from build123d import *

# Parameters (mm, degrees)
SKETCH_1_W             = 25
SKETCH_1_H             = 24
EXTRUDE_271_DEPTH      = 1
EXTRUDE_458_DEPTH      = 3.8
SKETCH_3_W             = 22
SKETCH_3_H             = 4.802295703
EXTRUDE_725_DEPTH      = 1.5
HOLE_WIZARD_886_D      = 0.5
HOLE_WIZARD_886_DEPTH  = 1
HOLE_WIZARD_1548_D     = 2
HOLE_WIZARD_1548_DEPTH = 16.4


with BuildPart() as part:
    # Эскиз1 → Extrude 271 (new body)
    with BuildSketch(Plane(origin=(0, 0, -1), x_dir=(-1, 0, 0), z_dir=(0, 0, -1))):
        with Locations((-12.5, 12)):
            Rectangle(SKETCH_1_W, SKETCH_1_H)
    extrude(amount=-EXTRUDE_271_DEPTH)

    # Эскиз2 → Extrude 458 (add)
    with BuildSketch(Plane(origin=(0, 0, -1), x_dir=(-1, 0, 0), z_dir=(0, 0, -1))):
        with BuildLine():
            Line((-5.95, 10.75), (-3.949995117, 10.75))
            ThreePointArc((-3.949995117, 10.75), (-1.949995117, 8.75), (-3.949995117, 6.75))
            Line((-3.949995117, 6.75), (-5.95, 6.75))
            Line((-5.95, 6.75), (-5.95, 2.2))
            Line((-5.95, 2.2), (-19.05, 2.2))
            Line((-19.05, 2.2), (-19.05, 6.75))
            Line((-19.05, 6.75), (-21.050009766, 6.75))
            ThreePointArc((-21.050009766, 6.75), (-23.050009766, 8.75), (-21.050009766, 10.75))
            Line((-21.050009766, 10.75), (-19.05, 10.75))
            Line((-19.05, 10.75), (-19.05, 15.3))
            Line((-19.05, 15.3), (-5.95, 15.3))
            Line((-5.95, 15.3), (-5.95, 10.75))
        make_face()
    extrude(amount=EXTRUDE_458_DEPTH)

    # Эскиз3 → Extrude 725 (add)
    with BuildSketch(Plane(origin=(0, 0, -1), x_dir=(-1, 0, 0), z_dir=(0, 0, -1))):
        with Locations((-12.5, 21.098852149)):
            Rectangle(SKETCH_3_W, SKETCH_3_H)
    extrude(amount=EXTRUDE_725_DEPTH)

    # Эскиз4 → Revolve 834 (revolve)
    with BuildSketch(Plane.XZ.offset(-8.75), mode=Mode.PRIVATE) as revolve_834_sk:
        Polygon((19.1, -4.8), (12.5, -4.8), (12.5, -16.4), (19.5, -16.4), (19.5, -13.3), (18.25, -13.3), (18.25, -9.3), (19.1, -9.3), align=None)
    revolve(revolve_834_sk.sketch.rotate(Axis((12.5, 8.75, -4.8), (0, 0, -1)), 180), axis=Axis((12.5, 8.75, -4.8), (0, 0, -1)))

    # Hole Wizard 886
    with Locations(Plane.XY):
        with Locations((12.5, 8.75)):
            Hole(HOLE_WIZARD_886_D / 2, depth=HOLE_WIZARD_886_DEPTH)

    # Hole Wizard 1548
    with Locations(Plane.XY):
        with Locations((2, 2), (2, 15.5), (23, 15.5), (23, 2)):
            Hole(HOLE_WIZARD_1548_D / 2, depth=HOLE_WIZARD_1548_DEPTH)


solid = part.part
CAD build for the part. Positions are in the model's coordinates, mm. A direction names the side the tool comes from. Coordinates: 2 decimals unless noted, no trailing zeros. Write each loop counter-clockwise with the first axis right and the second up, starting at its lowest first coordinate (ties: lowest second). Pieces come first, ordered by that corner, then holes. Notation, with made-up numbers: (-34.75, 59.5) - (10.25, 59.5) arc R21 cw to (10.25, 66.5) - close; hole circle Ø5 at (63.25, 84). An arc over 180 degrees is marked (long way). Use a Markdown table: item, result. Add a question column.
Item 1: Mould opens along Z. For faces 5 (the face through (8.952, 14.315, -7.018)), 6 (the face through (23.217, 14.524, -0.507)) say: pulls with the +Z half, pulls with the -Z half, needs draft (parallel to the pull), parting line crosses it, or undercut.
Item 2: Drill centre lines: L1, parallel to Y at x = 23, z = -0.6; L2, parallel to Z at x = 15.5, y = 2.75; L3, parallel to Z at x = 17, y = 13.5. Where is each one in solid material? Low to high. Write a range as from..to.
Item 3: Flat gauge pins, fed straight in: pin 1 (3 mm diameter, centred on y = 4.5, z = -3.5, fed in from -X); pin 2 (2 mm diameter, centred on x = 7, z = -11.5, fed in from +Y); pin 3 (1.1 mm diameter, centred on y = 14, z = -3, fed in from +X); pin 4 (1.6 mm diameter, centred on x = 2, y = 2, fed in from -Z). Where does each tip first touch, or does it go through?
Item 4: Band-saw the part on B-B, the plane x = 17.25. Give the cut face in (y, z), and give its area (3 significant figures).
Item 5: 3-axis set-ups, long thin cutter, end or side, ignore diameter. For faces 1 (the face through (13, 15, -9.3)), 2 (the face through (1.95, 8.79, -2.87)), 3 (the face through (23.5, 21, -2)), 4 (the face through (13, 18.698, -2)): which of +Z, -Z, +X, -X, +Y, -Y reach the whole face in a straight line?
Item 6: Band-saw the part on C-C, the plane z = -15.5. Give the cut face in (x, y).
Item 7: Band-saw the part on A-A, the plane x = 22.5. Give the cut face in (y, z), and give its area (3 significant figures).
Numbers:
| question | item | result |
|---|---|---|
| 1 | face 5 | undercut |
| 1 | face 6 | needs draft |
| 2 | L1 | 0..1, 3..14.5, 16.5..24 |
| 2 | L2 | -16.4..-13.3, -4.8..0 |
| 2 | L3 | -16.4..-13.3, -9.3..0 |
| 3 | pin 1 | x = 5.95 |
| 3 | pin 2 | y = 12.33 |
| 3 | pin 3 | x = 19.05 |
| 3 | pin 4 | through |
| 4 | outline | (0, -1) - (2.2, -1) - (2.2, -4.8) - (4.17, -4.8) - (4.17, -9.3) - (5.51, -9.3) - (5.51, -13.3) - (3.61, -13.3) - (3.61, -16.4) - (13.89, -16.4) - (13.89, -13.3) - (11.99, -13.3) - (11.99, -9.3) - (13.33, -9.3) - (13.33, -4.8) - (15.3, -4.8) - (15.3, -1) - (18.7, -1) - (18.7, -2.5) - (23.5, -2.5) - (23.5, -1) - (24, -1) - (24, 0) - (0, 0) - close |
| 4 | area | 180 mm2 |
| 5 | face 1 | none |
| 5 | face 2 | -Z, -X |
| 5 | face 3 | -Z, +X, +Y, -Y |
| 5 | face 4 | -Z, +X, -X |
| 6 | outline | circle Ø14 at (12.5, 8.75) |
| 7 | outline | (0, -1) - (1.13, -1) - (1.13, 0) - (0, 0) - close; (2.87, -1) - (7.37, -1) - (7.37, -4.8) - (10.13, -4.8) - (10.13, -1) - (14.63, -1) - (14.63, 0) - (2.87, 0) - close; (16.37, -1) - (18.7, -1) - (18.7, -2.5) - (23.5, -2.5) - (23.5, -1) - (24, -1) - (24, 0) - (16.37, 0) - close |
| 7 | area | 38.2 mm2 |
